from build123d import *

# Parameters (mm, degrees)
SKETCH1_W               = 146.36
SKETCH1_H               = 101.6
BOSS_EXTRUDE1_DEPTH     = 3.18
CUT_EXTRUDE1_START      = -4.18
SKETCH2_W               = 3.18
SKETCH2_H               = 20
SKETCH2_W_2             = 13
SKETCH2_H_2             = 3
SKETCH2_W_3             = 2.82
SKETCH2_H_3             = 7
CUT_EXTRUDE1_DEPTH      = 5.18
CUT_EXTRUDE2_START      = -4.18
SKETCH3_W               = 63.305
SKETCH3_H               = 3.18
CUT_EXTRUDE2_DEPTH      = 5.18
SKETCH4_R               = 1.55
CUT_EXTRUDE3_DEPTH      = 1
CUT_EXTRUDE3_DEPTH_BACK = 4.18


with BuildPart() as part:
    # Sketch1 → Boss-Extrude1 (new body)
    with BuildSketch(Plane.XY):
        Rectangle(SKETCH1_W, SKETCH1_H)
    extrude(amount=BOSS_EXTRUDE1_DEPTH)

    # Sketch2 → Cut-Extrude1 (cut)
    with BuildSketch(Plane.XY.offset(3.18).offset(CUT_EXTRUDE1_START)):
        with Locations((-71.59, 0)):
            Rectangle(SKETCH2_W, SKETCH2_H)
        with Locations((-66.68, 0)):
            Rectangle(SKETCH2_W_2, SKETCH2_H_2)
        with Locations((-64.59, 0)):
            Rectangle(SKETCH2_W_3, SKETCH2_H_3)
    cut_extrude1 = extrude(amount=CUT_EXTRUDE1_DEPTH, mode=Mode.SUBTRACT)

    # Mirror1: Cut-Extrude1 across plane
    add(cut_extrude1.mirror(Plane(origin=(0, 0, 0), x_dir=(0, 0, 1), z_dir=(1, 0, 0))), mode=Mode.SUBTRACT)

    # Sketch3 → Cut-Extrude2 (cut)
    with BuildSketch(Plane.XY.offset(3.18).offset(CUT_EXTRUDE2_START)):
        with Locations((-41.5275, -49.21)):
            Rectangle(SKETCH3_W, SKETCH3_H)
    cut_extrude2 = extrude(amount=CUT_EXTRUDE2_DEPTH, mode=Mode.SUBTRACT)

    # Mirror2: Cut-Extrude2 across plane
    add(cut_extrude2.mirror(Plane(origin=(0, 0, 0), x_dir=(0, 0, 1), z_dir=(1, 0, 0))), mode=Mode.SUBTRACT)

    # Sketch4 → Cut-Extrude3 (cut, two sides)
    with BuildSketch(Plane.XY.offset(3.18)) as cut_extrude3_sk:
        with Locations((0, -48.8)):
            Circle(SKETCH4_R)
    extrude(amount=CUT_EXTRUDE3_DEPTH, mode=Mode.SUBTRACT)
    extrude(cut_extrude3_sk.sketch, amount=-CUT_EXTRUDE3_DEPTH_BACK, mode=Mode.SUBTRACT)


solid = part.part
Check sheet for the modelled part. Datum: model origin and axes. Units: mm. A direction names the side the tool comes from. Round coordinates to 2 decimals unless told otherwise and drop trailing zeros. Order: outer loops, then holes, each group sorted by start corner. A loop starts at its lowest first (then second) coordinate and runs counter-clockwise, first axis right, second up.
(1) Cross-section at A-A, the plane x = 0. Enter the section's corners in (y, z), and give its area (3 significant figures).
(2) Go/stop test with flat-tipped pins: P1, Ø1, axis at y = -49.5, z = 2, coming from the +X side (3 decimals); P2, Ø1, axis at y = -2.5, z = 1.5, coming from the -X side; P3, Ø0.6, axis at y = -2, z = 2, coming from the +X side. Record where each tip stops, or that it passes through.
(3) Draft check along Y on faces 1 (the flat face through (60.18, 0, 2)), 2 (the flat face through (-73.18, 30, 2)), 3 (the flat face through (42, -47.62, 2)). Enter one of: pulls with the +Y half, pulls with the -Y half, needs draft (parallel to the pull), parting line crosses it, or undercut.
(4) Access from +Z, -Z, +X, -X, +Y, -Y to the whole of each face (thin tool, end or side, straight path). Record for faces 4 (the flat face through (68, 1.5, 2)), 5 (the flat face through (-65, -3.5, 2)), 6 (the flat face through (-9.875, -49, 2)), 7 (the flat face through (-72, -10, 2)).
(5) Scan lines: probe 1 along Y at (x, z) = (-64.5, 2.2); probe 2 along Y at (x, z) = (0, 1.1); probe 3 along Y at (x, z) = (-57, 1.5). Record each from-to range of solid material in increasing order.
(6) Cross-section at B-B, the plane x = -46.5. Enter the section's corners in (y, z).
Check sheet entries:
1. outline: (-50.8, 0) - (-50.35, 0) - (-50.35, 3.18) - (-50.8, 3.18) - close; (-47.25, 0) - (50.8, 0) - (50.8, 3.18) - (-47.25, 3.18) - close
1. area: 313 mm2
2. P1: stops at x = 9.875
2. P2: stops at x = -70
2. P3: stops at x = 70
3. face 1: undercut
3. face 2: needs draft
3. face 3: pulls with the -Y half
4. face 4: +Z, -Z, +X
4. face 5: +Z, -Z
4. face 6: +Z, -Z, -X, -Y
4. face 7: +Z, -Z, -X
5. probe 1: y = -47.62 to -3.5, 3.5 to 50.8
5. probe 2: y = -50.8 to -50.35, -47.25 to 50.8
5. probe 3: y = -47.62 to 50.8
6. outline: (-47.62, 0) - (50.8, 0) - (50.8, 3.18) - (-47.62, 3.18) - close
